Here's how the part is built. I have some questions about the finished solid (model axes, mm). Round coordinates to 2 decimals unless told otherwise and drop trailing zeros. Order: outer loops, then holes, each group sorted by start corner. A loop starts at its lowest first (then second) coordinate and runs counter-clockwise, first axis right, second up.
```python
from build123d import *

# Parameters (mm, degrees)
F1_DEPTH = 8


with BuildPart() as f1:
    # F0 (on Top) → F1 (new body)
    with BuildSketch(Plane.XY):
        with BuildLine():
            ThreePointArc((-3.561162, 5.021676), (-8.002963, 2.864677), (-5.868373, -1.587937))
            ThreePointArc((-5.868373, -1.587937), (-5.350405, -6.807139), (-0.147566, -6.144698))
            ThreePointArc((-0.147566, -6.144698), (5.002213, -7.073285), (5.826574, -1.905798))
            ThreePointArc((5.826574, -1.905798), (8.176987, 2.66641), (3.560513, 4.928642))
            ThreePointArc((3.560513, 4.928642), (0.046518, 8.560924), (-3.561162, 5.021676))
        make_face()
        with BuildLine():
            ThreePointArc((-4.77668, -1.477608), (-4.805196, -1.382061), (-4.831801, -1.285963))
            ThreePointArc((-4.831801, -1.285963), (-7.516984, 2.73769), (-2.873108, 4.092096))
            ThreePointArc((-2.873108, 4.092096), (-2.867466, 4.096052), (-2.861818, 4.1))
            ThreePointArc((-2.861818, 4.1), (0, 8), (2.861818, 4.1))
            ThreePointArc((2.861818, 4.1), (2.943989, 4.041402), (3.024962, 3.981156))
            ThreePointArc((3.024962, 3.981156), (7.61462, 2.453073), (4.780023, -1.466757))
            ThreePointArc((4.780023, -1.466757), (4.742433, -1.584087), (4.701962, -1.700456))
            ThreePointArc((4.701962, -1.700456), (4.611728, -6.536969), (0.025059, -4.999937))
            ThreePointArc((0.025059, -4.999937), (-0.11752, -4.998619), (-0.260004, -4.993235))
            ThreePointArc((-0.260004, -4.993235), (-4.913838, -6.313018), (-4.77668, -1.477608))
        make_face(mode=Mode.SUBTRACT)
    extrude(amount=F1_DEPTH)


solid = f1.part
```
1. If we section it at C-C, the plane x = -6.5: Write out the boundary of the cut face in (y, z), and give its area (3 significant figures).
Evaluation:
outline: (-5.22, 0) - (-2.67, 0) - (-2.67, 8) - (-5.22, 8) - close; (-1.29, 0) - (-0.69, 0) - (-0.69, 8) - (-1.29, 8) - close; (4.11, 0) - (4.71, 0) - (4.71, 8) - (4.11, 8) - close
area: 30.0 mm2
2. I'm going to push a flat-ended pin straight in: P1, Ø4, axis at y = -1, z = 6, coming from the -X side. Where does the tip first touch, or does it pass through?
Evaluation:
P1: stops at x = -8.13
3. If we mould it in two halves opening along Y, with no side actions, what happens to faces 1 (the flat face through (0, -6, 8)), 2 (the cylindrical face through (0, 8, 4))? For each: released by +Y, released by -Y, zero draft, split by the parting line, or undercut.
Evaluation:
face 1: zero draft
face 2: undercut
4. If we section it at B-B, the plane y = 0.5: Write out the boundary of the cut face in (x, z), and give its area (3 significant figures).
Evaluation:
outline: (-7.98, 0) - (-7.44, 0) - (-7.44, 8) - (-7.98, 8) - close; (7.58, 0) - (8.21, 0) - (8.21, 8) - (7.58, 8) - close
area: 9.38 mm2
5. I need wall thicknesses on probe 1 along Y at (x, z) = (5.5, 5.5); probe 2 along X at (y, z) = (-6.5, 5.75); probe 3 along X at (y, z) = (0, 4.5). Which ranges of each line are inside material? Lowest first, please.
Evaluation:
probe 1: y = -6.65 to -5.55, -2.62 to -1.37, 4.44 to 5.06
probe 2: x = -5.69 to -4.64, -1.5 to -0.45, 0.13 to 1.1, 4.66 to 5.64
probe 3: x = -7.75 to -7.16, 7.34 to 8.02
6. If we section it at A-A, the plane x = 7.25: Write out the boundary of the cut face in (y, z), and give its area (3 significant figures).
Evaluation:
outline: (-1.07, 0) - (-0.14, 0) - (-0.14, 8) - (-1.07, 8) - close; (3.21, 0) - (4.13, 0) - (4.13, 8) - (3.21, 8) - close
area: 14.9 mm2
